```python
from build123d import *

# Parameters (mm, degrees)
SKETCH1_R           = 15
SKETCH1_R_2         = 5
BOSS_EXTRUDE2_DEPTH = 20
SKETCH7_OUTSIDE_W   = 203.058
SKETCH7_OUTSIDE_H   = 184.494
CUT_EXTRUDE4_DEPTH  = 4
CUT_EXTRUDE5_DEPTH  = 4


with BuildPart() as part:
    # Sketch1 → Boss-Extrude2 (new body)
    with BuildSketch(Plane.XY):
        with BuildLine():
            Line((-9.952202212, -80.976560871), (-15.609727063, -23.320317388))
            ThreePointArc((-15.609727063, -23.320317388), (-19.485571585, -11.25), (-28.000850814, -1.858261489))
            Line((-28.000850814, -1.858261489), (-75.103859931, 31.869420496))
            ThreePointArc((-75.103859931, 31.869420496), (-77.942286341, 45), (-65.151657719, 49.107140374))
            Line((-65.151657719, 49.107140374), (-12.391123751, 25.178578877))
            ThreePointArc((-12.391123751, 25.178578877), (0, 22.5), (12.391123751, 25.178578877))
            Line((12.391123751, 25.178578877), (65.151657719, 49.107140374))
            ThreePointArc((65.151657719, 49.107140374), (77.942286341, 45), (75.103859931, 31.869420496))
            Line((75.103859931, 31.869420496), (28.000850814, -1.858261489))
            ThreePointArc((28.000850814, -1.858261489), (19.485571585, -11.25), (15.609727063, -23.320317388))
            Line((15.609727063, -23.320317388), (9.952202212, -80.976560871))
            ThreePointArc((9.952202212, -80.976560871), (0, -90), (-9.952202212, -80.976560871))
        make_face()
        Circle(SKETCH1_R, mode=Mode.SUBTRACT)
        with Locations((0, -80)):
            Circle(SKETCH1_R_2, mode=Mode.SUBTRACT)
        with Locations((-69.282032303, 40)):
            Circle(SKETCH1_R_2, mode=Mode.SUBTRACT)
        with Locations((69.282032303, 40)):
            Circle(SKETCH1_R_2, mode=Mode.SUBTRACT)
    extrude(amount=BOSS_EXTRUDE2_DEPTH)

    # Sketch7 outside → Cut-Extrude4 (cut)
    with BuildSketch(Plane.XY.offset(20)):
        with Locations((0, -20)):
            Rectangle(SKETCH7_OUTSIDE_W, SKETCH7_OUTSIDE_H)
        with BuildLine():
            Line((-15.609727063, -23.320317388), (-9.952202212, -80.976560871))
            ThreePointArc((-9.952202212, -80.976560871), (0, -90), (9.952202212, -80.976560871))
            Line((9.952202212, -80.976560871), (15.609727063, -23.320317388))
            ThreePointArc((15.609727063, -23.320317388), (19.485571585, -11.25), (28.000850814, -1.858261489))
            Line((28.000850814, -1.858261489), (75.103859931, 31.869420496))
            ThreePointArc((75.103859931, 31.869420496), (77.942286341, 45), (65.151657719, 49.107140374))
            Line((65.151657719, 49.107140374), (12.391123751, 25.178578877))
            ThreePointArc((12.391123751, 25.178578877), (0, 22.5), (-12.391123751, 25.178578877))
            Line((-12.391123751, 25.178578877), (-65.151657719, 49.107140374))
            ThreePointArc((-65.151657719, 49.107140374), (-77.942286341, 45), (-75.103859931, 31.869420496))
            Line((-75.103859931, 31.869420496), (-28.000850814, -1.858261489))
            ThreePointArc((-28.000850814, -1.858261489), (-19.485571585, -11.25), (-15.609727063, -23.320317388))
        make_face(mode=Mode.SUBTRACT)
        with BuildLine():
            Line((-25.609534097, 2.579081047), (-62.746066413, 29.170357813))
            ThreePointArc((-62.746066413, 29.170357813), (-63.580283737, 30.721196932), (-62.865089457, 32.330394762))
            ThreePointArc((-62.865089457, 32.330394762), (-60.621778265, 35), (-59.431487906, 38.2775671))
            ThreePointArc((-59.431487906, 38.2775671), (-58.395478846, 39.70154243), (-56.63530411, 39.754508595))
            Line((-56.63530411, 39.754508595), (-15.038316754, 20.888966584))
            ThreePointArc((-15.038316754, 20.888966584), (-12.749228932, 17.929225173), (-13.908722156, 14.371758695))
            ThreePointArc((-13.908722156, 14.371758695), (-17.320508076, 10), (-19.400669205, 4.859427374))
            ThreePointArc((-19.400669205, 4.859427374), (-21.901778936, 2.076543547), (-25.609534097, 2.579081047))
        make_face()
        with BuildLine():
            Line((25.609534097, 2.579081047), (62.746066413, 29.170357813))
            ThreePointArc((62.746066413, 29.170357813), (63.580283737, 30.721196932), (62.865089457, 32.330394762))
            ThreePointArc((62.865089457, 32.330394762), (60.621778265, 35), (59.431487906, 38.2775671))
            ThreePointArc((59.431487906, 38.2775671), (58.395478846, 39.70154243), (56.63530411, 39.754508595))
            Line((56.63530411, 39.754508595), (15.038316754, 20.888966584))
            ThreePointArc((15.038316754, 20.888966584), (12.749228932, 17.929225173), (13.908722156, 14.371758695))
            ThreePointArc((13.908722156, 14.371758695), (17.320508076, 10), (19.400669205, 4.859427374))
            ThreePointArc((19.400669205, 4.859427374), (21.901778936, 2.076543547), (25.609534097, 2.579081047))
        make_face()
        with BuildLine():
            Line((-10.571217344, -23.468047631), (-6.110762303, -68.924866408))
            ThreePointArc((-6.110762303, -68.924866408), (-5.184804891, -70.422739362), (-3.43360155, -70.607961862))
            ThreePointArc((-3.43360155, -70.607961862), (0, -70), (3.43360155, -70.607961862))
            ThreePointArc((3.43360155, -70.607961862), (5.184804891, -70.422739362), (6.110762303, -68.924866408))
            Line((6.110762303, -68.924866408), (10.571217344, -23.468047631))
            ThreePointArc((10.571217344, -23.468047631), (9.152550004, -20.00576872), (5.491947049, -19.231186069))
            ThreePointArc((5.491947049, -19.231186069), (0, -20), (-5.491947049, -19.231186069))
            ThreePointArc((-5.491947049, -19.231186069), (-9.152550004, -20.00576872), (-10.571217344, -23.468047631))
        make_face()
    extrude(amount=-CUT_EXTRUDE4_DEPTH, mode=Mode.SUBTRACT)

    # Sketch3 → Cut-Extrude5 (cut)
    with BuildSketch(Plane(origin=(0, 0, 0), x_dir=(-1, 0, 0), z_dir=(0, 0, -1))):
        with BuildLine():
            Line((10.571217344, -23.468047631), (6.110762303, -68.924866408))
            ThreePointArc((6.110762303, -68.924866408), (5.184804891, -70.422739362), (3.43360155, -70.607961862))
            ThreePointArc((3.43360155, -70.607961862), (0, -70), (-3.43360155, -70.607961862))
            ThreePointArc((-3.43360155, -70.607961862), (-5.184804891, -70.422739362), (-6.110762303, -68.924866408))
            Line((-6.110762303, -68.924866408), (-10.571217344, -23.468047631))
            ThreePointArc((-10.571217344, -23.468047631), (-9.152550004, -20.00576872), (-5.491947049, -19.231186069))
            ThreePointArc((-5.491947049, -19.231186069), (0, -20), (5.491947049, -19.231186069))
            ThreePointArc((5.491947049, -19.231186069), (9.152550004, -20.00576872), (10.571217344, -23.468047631))
        make_face()
        with BuildLine():
            Line((-25.609534097, 2.579081047), (-62.746066413, 29.170357813))
            ThreePointArc((-62.746066413, 29.170357813), (-63.580283737, 30.721196932), (-62.865089457, 32.330394762))
            ThreePointArc((-62.865089457, 32.330394762), (-60.621778265, 35), (-59.431487906, 38.2775671))
            ThreePointArc((-59.431487906, 38.2775671), (-58.395478846, 39.70154243), (-56.63530411, 39.754508595))
            Line((-56.63530411, 39.754508595), (-15.038316754, 20.888966584))
            ThreePointArc((-15.038316754, 20.888966584), (-12.749228932, 17.929225173), (-13.908722156, 14.371758695))
            ThreePointArc((-13.908722156, 14.371758695), (-17.320508076, 10), (-19.400669205, 4.859427374))
            ThreePointArc((-19.400669205, 4.859427374), (-21.901778936, 2.076543547), (-25.609534097, 2.579081047))
        make_face()
        with BuildLine():
            Line((15.038316754, 20.888966584), (56.63530411, 39.754508595))
            ThreePointArc((56.63530411, 39.754508595), (58.395478846, 39.70154243), (59.431487906, 38.2775671))
            ThreePointArc((59.431487906, 38.2775671), (60.621778265, 35), (62.865089457, 32.330394762))
            ThreePointArc((62.865089457, 32.330394762), (63.580283737, 30.721196932), (62.746066413, 29.170357813))
            Line((62.746066413, 29.170357813), (25.609534097, 2.579081047))
            ThreePointArc((25.609534097, 2.579081047), (21.901778936, 2.076543547), (19.400669205, 4.859427374))
            ThreePointArc((19.400669205, 4.859427374), (17.320508076, 10), (13.908722156, 14.371758695))
            ThreePointArc((13.908722156, 14.371758695), (12.749228932, 17.929225173), (15.038316754, 20.888966584))
        make_face()
    extrude(amount=-CUT_EXTRUDE5_DEPTH, mode=Mode.SUBTRACT)


solid = part.part
```
Source: CAD feature listing. Evaluate the final solid. Frame: model axes, mm. A direction names the side the tool comes from. Coordinates: 2 decimals unless noted, no trailing zeros. Loops run counter-clockwise (first coordinate to the right, second up) from the corner with the lowest first, then second, coordinate; pieces in that order, holes last. Notation, with made-up numbers: (-22.75, 33.25) -> (5.25, 33.25) arc R30 cw to (5.25, 62.25) -> close; hole circle Ø5 at (43, -23.5). An arc over 180 degrees is marked (long way). One line per item, written item: value. Start each with the question number.
Q1. Section query A-A, the plane z = 13.75. Return the cut outline in (x, y), and give its area (3 significant figures).
Q2. Section query C-C, the plane y = 0. Return the cut outline in (x, z), and give its area (3 significant figures).
Q3. Section query D-D, the plane y = -62. Return the cut outline in (x, z).
Q4. Line query: line 1 along Y through (x, z) = (0, 12.5); line 2 along X through (y, z) = (44, 7.25); line 3 along Y through (x, z) = (-6.5, 8). Output: solid intervals per line, ascending.
Q5. Mould query, pull axis Y, two halves, no side actions, for faces 1 (the face through (12.76, 17.98, 18.03)), 2 (the face through (0, -90, 10)). Classes: pulls with the +Y half, pulls with the -Y half, needs draft (parallel to the pull), parting line crosses it, or undercut.
Q6. Contact query for flat-ended pins moving along their axis: P1, Ø4, axis at x = 0, y = -46, coming from the +Z side; P2, Ø3, axis at y = 11.5, z = 15.5, coming from the -X side; P3, Ø10, axis at x = 49.5, z = 12.5, coming from the -Y side. Output: stop coordinate, or through.
Q7. Set-up query: faces 3 (the face through (0, -45, 16)), 4 (the face through (-35.55, 30.19, 1.97)), 5 (the face through (-14.985, 0.66, 9.86)). Return all of +Z, -Z, +X, -X, +Y, -Y with unobstructed straight access to the full face (end or side cutting, diameter ignored); none if empty.
Q8. Section query B-B, the plane x = 0. Return the cut outline in (y, z).
Results:
1. outline: (-75.1, 31.87) -> (-28, -1.86) arc R30 cw to (-15.61, -23.32) -> (-9.95, -80.98) arc R10 ccw to (9.95, -80.98) -> (15.61, -23.32) arc R30 cw to (28, -1.86) -> (75.1, 31.87) arc R10 ccw to (65.15, 49.11) -> (12.39, 25.18) arc R30 cw to (-12.39, 25.18) -> (-65.15, 49.11) arc R10 ccw to start; hole circle Ø10 at (-69.28, 40); hole circle Ø30 at (0, 0); hole circle Ø10 at (0, -80); hole circle Ø10 at (69.28, 40)
1. area: 5,790 mm^2
2. outline: (-30.6, 0) -> (-15, 0) -> (-15, 20) -> (-30.6, 20) -> close; (15, 0) -> (30.6, 0) -> (30.6, 20) -> (15, 20) -> close
2. area: 624 mm^2
3. outline: (-11.81, 0) -> (-6.79, 0) -> (-6.79, 4) -> (6.79, 4) -> (6.79, 0) -> (11.81, 0) -> (11.81, 20) -> (6.79, 20) -> (6.79, 16) -> (-6.79, 16) -> (-6.79, 20) -> (-11.81, 20) -> close
4. line 1: -90 to -85, -75 to -15, 15 to 22.5
4. line 2: -78.45 to -72.28, -66.28 to -53.89, 53.89 to 66.28, 72.28 to 78.45
4. line 3: -87.6 to -13.52, 13.52 to 23.21
5. face 1: undercut
5. face 2: pulls with the -Y half
6. P1: z = 16
6. P2: x = -48.75
6. P3: y = 9.96
7. face 3: +Z
7. face 4: -Z
7. face 5: +Z, -Z
8. outline: (-90, 0) -> (-85, 0) -> (-85, 20) -> (-90, 20) -> close; (-75, 0) -> (-70, 0) -> (-70, 4) -> (-20, 4) -> (-20, 0) -> (-15, 0) -> (-15, 20) -> (-20, 20) -> (-20, 16) -> (-70, 16) -> (-70, 20) -> (-75, 20) -> close; (15, 0) -> (22.5, 0) -> (22.5, 20) -> (15, 20) -> close
